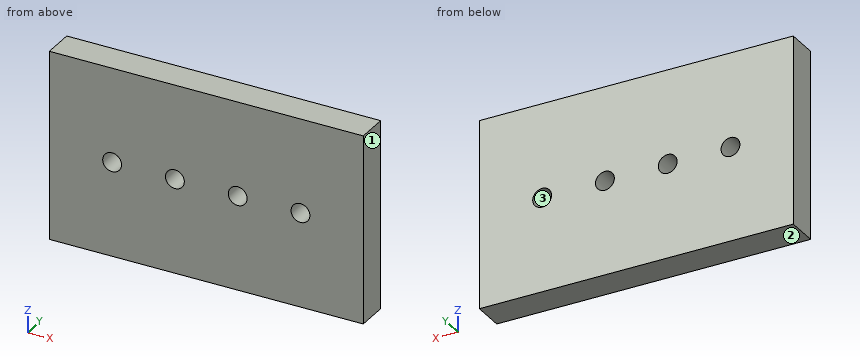
from build123d import *

# Parameters (mm, degrees)
SKETCH_1_W             = 100
SKETCH_1_H             = 60
EXTRUDE_1_DEPTH        = 10
SKETCH_2_R             = 3
CUT_EXTRUDE_1_DEPTH    = 20
PATTERN_LINEAR_1_COUNT = 4
PATTERN_LINEAR_1_PITCH = 20


with BuildPart() as part:
    # 草图1 → 凸台-拉伸1 (new body)
    with BuildSketch(Plane(origin=(0, 0, 0), x_dir=(1, 0, 0), z_dir=(0, 1, 0))):
        Rectangle(SKETCH_1_W, SKETCH_1_H)
    extrude(amount=EXTRUDE_1_DEPTH)

    # 草图2 → 切除-拉伸1 (cut)
    with BuildSketch(Plane(origin=(0, 0, 0), x_dir=(1, 0, 0), z_dir=(0, 1, 0))):
        with Locations(Location((-30, 0, 0), (0, 0, 90))):
            Circle(SKETCH_2_R)
    cut_extrude_1 = extrude(amount=CUT_EXTRUDE_1_DEPTH, mode=Mode.SUBTRACT)

    # 阵列(线性)1: 切除-拉伸1 ×4
    with Locations(*[(i * PATTERN_LINEAR_1_PITCH, 0, 0) for i in range(1, PATTERN_LINEAR_1_COUNT)]):
        add(cut_extrude_1, mode=Mode.SUBTRACT)


solid = part.part
Read the model definition and answer for the solid it produces. Units are mm, in the model's axes. Face numbers are marked on the shaded views. Round coordinates to 2 decimals unless told otherwise and drop trailing zeros. Write each loop counter-clockwise with the first axis right and the second up, starting at its lowest first coordinate (ties: lowest second). Pieces come first, ordered by that corner, then holes. Notation, with made-up numbers: (29.5, 33) - (56.5, 33) arc R26 ccw to (56.5, 61) - close; hole circle Ø5 at (87, 6.5). An arc over 180 degrees is marked (long way). One line per question, with ' | ' between items. Start each with the question number.
1. For a pull along X with two mould halves and no side action, classify the marked faces 1, 2 and 3 as +X half, -X half, draft (parallel to the pull), parting line (faces both ways), or undercut.
2. Find the intervals of material crossed by probe 1 along X at (y, z) = (5.5, 0); probe 2 along Z at (x, y) = (30, 5.75); probe 3 along X at (y, z) = (6.5, 2), in increasing order. Write a range as [from, to].
3. Section A-A (z = 0) is taken. Determine the outline of the cut face in (x, y).
4. Section C-C (x = -10) is taken. Determine the outline of the cut face in (y, z), and give its area (3 significant figures).
5. Section B-B (y = 8) is taken. Determine the outline of the cut face in (x, z), and give its area (3 significant figures).
Filled in:
1) face 1: +X half | face 2: draft | face 3: undercut
2) probe 1: [-50, -33], [-27, -13], [-7, 7], [13, 27], [33, 50] | probe 2: [-30, -3], [3, 30] | probe 3: [-50, -32.24], [-27.76, -12.24], [-7.76, 7.76], [12.24, 27.76], [32.24, 50]
3) outline: (-50, 0) - (-33, 0) - (-33, 10) - (-50, 10) - close; (-27, 0) - (-13, 0) - (-13, 10) - (-27, 10) - close; (-7, 0) - (7, 0) - (7, 10) - (-7, 10) - close; (13, 0) - (27, 0) - (27, 10) - (13, 10) - close; (33, 0) - (50, 0) - (50, 10) - (33, 10) - close
4) outline: (0, -30) - (10, -30) - (10, -3) - (0, -3) - close; (0, 3) - (10, 3) - (10, 30) - (0, 30) - close | area: 540 mm²
5) outline: (-50, -30) - (50, -30) - (50, 30) - (-50, 30) - close; hole circle Ø6 at (-30, 0); hole circle Ø6 at (-10, 0); hole circle Ø6 at (10, 0); hole circle Ø6 at (30, 0) | area: 5,890 mm²
